The listing builds one solid part. Answer for the finished solid, in the listing's coordinates (mm). A direction names the side the tool comes from. Give positions to 0.01 mm unless a question says otherwise; leave off trailing zeros. Write each loop counter-clockwise with the first axis right and the second up, starting at its lowest first coordinate (ties: lowest second). Pieces come first, ordered by that corner, then holes. Notation, with made-up numbers: M 44,18 L 53,18 A19 ccw 53,32 Z; hole C 76,7 d3. An arc over 180 degrees is marked long. Return JSON: item names as keys, results as strings.
from build123d import *

# Parameters (mm, degrees)
EXTRUDE_DEPTH    = 10
EXTRUDE001_DEPTH = 8


with BuildPart() as syringe_lock_bolt_hole_extrude:
    # Sketch002 → Extrude (new body)
    with BuildSketch(Plane.YZ):
        with BuildLine():
            Line((-1.8, -3.968126), (-1.8, 3.968126))
            ThreePointArc((1.8, 3.968126), (0, 5.768126), (-1.8, 3.968126))
            Line((1.8, 3.968126), (1.8, -3.968126))
            ThreePointArc((-1.8, -3.968126), (0, -5.768126), (1.8, -3.968126))
        make_face()
    extrude(amount=EXTRUDE_DEPTH)


with BuildPart() as syringe_lock_cut:
    # Sketch003 → Extrude001 (new body, symmetric)
    with BuildSketch(Plane.XZ):
        with BuildLine():
            Line((0.935284, -7.43412), (0, -5.199585))
            Line((0, -5.199585), (0, 5.375387))
            ThreePointArc((0, 5.375387), (-0.208788, 5.929256), (-0.731243, 6.207474))
            Line((-0.731243, 6.207474), (-3.352588, 6.54707))
            ThreePointArc((-3.952758, 7.230008), (-3.781394, 6.775418), (-3.352588, 6.54707))
            Line((-3.952758, 7.230008), (-3.952758, 7.667555))
            ThreePointArc((-3.086826, 8.533487), (-3.699132, 8.279861), (-3.952758, 7.667555))
            Line((-3.086826, 8.533487), (6.420806, 8.533487))
            ThreePointArc((6.987146, 7.967147), (6.821269, 8.36761), (6.420806, 8.533487))
            Line((6.987146, 7.967147), (6.987146, 7.416219))
            ThreePointArc((6.528064, 6.873501), (6.856982, 7.060797), (6.987146, 7.416219))
            Line((6.528064, 6.873501), (2.268866, 6.157352))
            ThreePointArc((2.268866, 6.157352), (1.880407, 5.936152), (1.726681, 5.516392))
            Line((1.726681, 5.516392), (1.726681, -7.527226))
            Line((1.726681, -7.527226), (0.935284, -7.43412))
        make_face()
    extrude(amount=EXTRUDE001_DEPTH, both=True)

    # Cut011: cut syringe lock bolt hole extrude
    add(syringe_lock_bolt_hole_extrude.part, mode=Mode.SUBTRACT)


with BuildPart() as syringe_lock_cut_1:
    # Cut011 placement: moved
    add(syringe_lock_cut.part.moved(Location((3.5, 43, 32))))


solid = syringe_lock_cut_1.part
Item 1: Given pin 1 Ø6 at (y, z) = (45, 32) entering from +X; pin 2 Ø5.5 at (y, z) = (46, 30) entering from -X, each flat-ended and moving along its own axis, determine where each tip first touches the part or whether it passes through.
Geometry results:
{"pin 1": "stops at x = 5.23", "pin 2": "stops at x = 3.5"}
Item 2: A cutting plane is placed at D-D, the plane z = 26.5. Write down the section's boundary in (x, y).
Geometry results:
{"outline": "M 3.63,35 L 5.23,35 L 5.23,42.05 L 3.63,42.05 Z; M 3.63,43.95 L 5.23,43.95 L 5.23,51 L 3.63,51 Z"}
Item 3: A cutting plane is placed at A-A, the plane z = 33. Write down the section's boundary in (x, y).
Geometry results:
{"outline": "M 3.5,35 L 5.23,35 L 5.23,41.2 L 3.5,41.2 Z; M 3.5,44.8 L 5.23,44.8 L 5.23,51 L 3.5,51 Z"}
Item 4: A cutting plane is placed at B-B, the plane y = 45.5. Write down the section's boundary in (x, z), plus the area to 3 significant figures.
Geometry results:
{"outline": "M -0.45,39.23 A0.69 ccw 0.15,38.55 L 2.77,38.21 A0.84 cw 3.5,37.38 L 3.5,26.8 L 4.44,24.57 L 5.23,24.47 L 5.23,37.52 A0.65 cw 5.77,38.16 L 10.03,38.87 A0.55 ccw 10.49,39.42 L 10.49,39.97 A0.57 ccw 9.92,40.53 L 0.41,40.53 A0.87 ccw -0.45,39.67 Z", "area": "45.6 mm2"}
Item 5: Which of the six approach directions +Z, -Z, +X, -X, +Y, -Y give full straight-line access (tool end or side, diameter ignored) to faces 1 (the flat face through (3.5, 48, 32)), 2 (the flat face through (5.227, 41, 31)), 3 (the cylindrical face through (4.351, 42.96, 26.232)), 4 (the cylindrical face through (4.376, 43.04, 37.768))?
Geometry results:
{"face 1": "-Z, -X, +Y, -Y", "face 2": "-Z, +X, +Y, -Y", "face 3": "+X, -X", "face 4": "+X"}
Item 6: Determine the mould class of faces 5 (the flat face through (5, 51, 36)), 6 (the cylindrical face through (3.3, 42.89, 37.92)), 7 (the flat face through (4, 41.2, 32)) for opening direction Z: +Z half, -Z half, draft (parallel to the pull), parting line (faces both ways), or undercut.
Geometry results:
{"face 5": "draft", "face 6": "-Z half", "face 7": "undercut"}
Item 7: A cutting plane is placed at C-C, the plane y = 43. Write down the section's boundary in (x, z), plus the area to 3 significant figures.
Geometry results:
{"outline": "M -0.45,39.23 A0.69 ccw 0.15,38.55 L 2.77,38.21 A0.84 cw 3.5,37.38 L 3.5,37.77 L 5.28,37.77 A0.65 cw 5.77,38.16 L 10.03,38.87 A0.55 ccw 10.49,39.42 L 10.49,39.97 A0.57 ccw 9.92,40.53 L 0.41,40.53 A0.87 ccw -0.45,39.67 Z; M 3.74,26.23 L 4.44,24.57 L 5.23,24.47 L 5.23,26.23 Z", "area": "25.7 mm2"}
Item 8: Find the intervals of material crossed by line 1 (Y direction, x = 5, z = 32.75); line 2 (X direction, y = 47.75, z = 31.75); line 3 (Z direction, x = 10, y = 36.5), in increasing order.
Geometry results:
{"line 1": "y = 35 to 41.2, 44.8 to 51", "line 2": "x = 3.5 to 5.23", "line 3": "z = 38.87 to 40.53"}
